```python
from build123d import *

# Parameters (mm, degrees)
BOSS_EXTRUDE1_DEPTH = 10
SKETCH2_R           = 2.5
CUT_EXTRUDE1_DEPTH  = 10
SKETCH3_R           = 11
CUT_EXTRUDE2_DEPTH  = 10
SKETCH4_R           = 2.5
CUT_EXTRUDE3_DEPTH  = 10


with BuildPart() as part:
    # Sketch1 → Boss-Extrude1 (new body)
    with BuildSketch(Plane(origin=(0, 0, 0), x_dir=(0, 0, -1), z_dir=(1, 0, 0))):
        with BuildLine():
            ThreePointArc((-209.31, 0), (0, -209.31), (209.31, 0))
            Line((209.31, 0), (-209.31, 0))
        make_face()
        with BuildLine():
            Line((-209.31, 0), (209.31, 0))
            ThreePointArc((209.31, 0), (0, 209.31), (-209.31, 0))
        make_face()
        with BuildLine():
            Line((-209.31, -224.4), (209.31, -224.4))
            Line((209.31, -224.4), (209.31, 0))
            ThreePointArc((209.31, 0), (0, -209.31), (-209.31, 0))
            Line((-209.31, 0), (-209.31, -224.4))
        make_face()
    extrude(amount=BOSS_EXTRUDE1_DEPTH)

    # Sketch2 → Cut-Extrude1 (cut)
    with BuildSketch(Plane(origin=(10, 0, 0), x_dir=(0, 0, -1), z_dir=(1, 0, 0))):
        with Locations((129.534891246, 129.534891246)):
            Circle(SKETCH2_R)
        with Locations((92.609775132, 92.609775132)):
            Circle(SKETCH2_R)
        with Locations((92.609775132, -92.609775132)):
            Circle(SKETCH2_R)
        with Locations((129.534891246, -129.534891246)):
            Circle(SKETCH2_R)
        with Locations((-92.609775132, -92.609775132)):
            Circle(SKETCH2_R)
        with Locations((-129.534891246, -129.534891246)):
            Circle(SKETCH2_R)
        with Locations((-92.609775132, 92.609775132)):
            Circle(SKETCH2_R)
        with Locations((-129.534891246, 129.534891246)):
            Circle(SKETCH2_R)
    extrude(amount=-CUT_EXTRUDE1_DEPTH, mode=Mode.SUBTRACT)

    # Sketch3 → Cut-Extrude2 (cut)
    with BuildSketch(Plane(origin=(10, 0, 0), x_dir=(0, 0, -1), z_dir=(1, 0, 0))):
        Circle(SKETCH3_R)
    extrude(amount=-CUT_EXTRUDE2_DEPTH, mode=Mode.SUBTRACT)

    # Sketch4 → Cut-Extrude3 (cut)
    with BuildSketch(Plane(origin=(10, 0, 0), x_dir=(0, 0, -1), z_dir=(1, 0, 0))):
        with Locations((-151.806215462, 102.53511129)):
            Circle(SKETCH4_R)
        with Locations(Location((-102.53511129, 151.806215462, 0), (0, 0, 180))):
            Circle(SKETCH4_R)
        with Locations((102.53511129, 151.806215462)):
            Circle(SKETCH4_R)
        with Locations(Location((151.806215462, 102.53511129, 0), (0, 0, 180))):
            Circle(SKETCH4_R)
        with Locations((151.806215462, -102.53511129)):
            Circle(SKETCH4_R)
        with Locations(Location((102.53511129, -151.806215462, 0), (0, 0, 180))):
            Circle(SKETCH4_R)
        with Locations((-102.53511129, -151.806215462)):
            Circle(SKETCH4_R)
        with Locations(Location((-151.806215462, -102.53511129, 0), (0, 0, 180))):
            Circle(SKETCH4_R)
    extrude(amount=-CUT_EXTRUDE3_DEPTH, mode=Mode.SUBTRACT)


solid = part.part
```
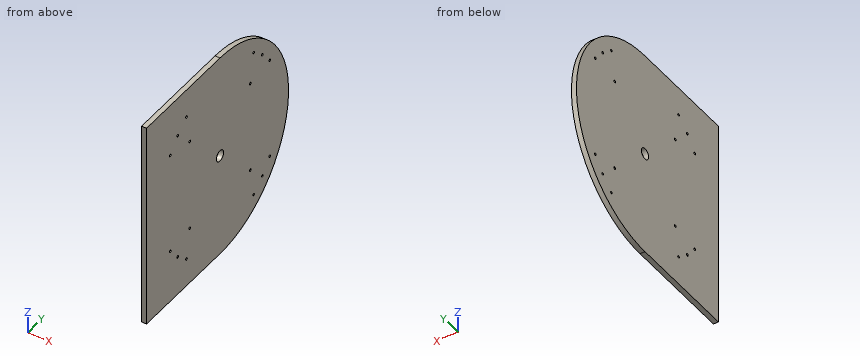
Geometry check sheet. Reference: the model listing, model coordinates, mm. Give positions to 0.01 mm unless a question says otherwise; leave off trailing zeros. Write each loop counter-clockwise with the first axis right and the second up, starting at its lowest first coordinate (ties: lowest second). Pieces come first, ordered by that corner, then holes. Notation, with made-up numbers: (30.5, 54.25) - (88.5, 54.25) arc R20 ccw to (88.5, 89.25) - close; hole circle Ø1 at (46, 59.25). An arc over 180 degrees is marked (long way). Use a Markdown table: item, result.
Q1. Section check A-A, the plane z = 0. Enter the section's corners in (x, y).
Computed:
| item | result |
|---|---|
| outline | (0, -224.4) - (10, -224.4) - (10, -11) - (0, -11) - close; (0, 11) - (10, 11) - (10, 209.31) - (0, 209.31) - close |
Q2. Go/stop test with flat-tipped pins: P1, Ø8, axis at y = -151.81, z = 102.54, coming from the -X side; P2, Ø1, axis at x = 8, y = 94.5, coming from the -Z side; P3, Ø2, axis at x = 1.5, y = 82, coming from the +Z side; P4, Ø5, axis at x = 4, y = 101, coming from the -Z side. Record where each tip stops, or that it passes through.
Computed:
| item | result |
|---|---|
| P1 | stops at x = 0 |
| P2 | stops at z = -187.02 |
| P3 | stops at z = 193 |
| P4 | stops at z = -184.68 |
Q3. Thickness scan on L1, parallel to Y at x = 8.25, z = 128; L2, parallel to Z at x = 8.25, y = -94.5; L3, parallel to Z at x = 8.5, y = 9. Record the ranges inside material, lowest first. Write a range as [from, to].
Computed:
| item | result |
|---|---|
| L1 | y = [-224.4, -131.51], [-127.56, 127.56], [131.51, 165.61] |
| L2 | z = [-209.31, -94.25], [-90.97, 90.97], [94.25, 209.31] |
| L3 | z = [-209.12, -6.32], [6.32, 209.12] |
Q4. Section check B-B, the plane x = 8.5. Give the number of separate pieces and of enclosed holes in the cut face, then the cut area to 3 significant figures.
Computed:
| item | result |
|---|---|
| separate pieces | 1 |
| enclosed holes | 17 |
| area | 162,000 mm² |
Q5. Section check C-C, the plane y = 117.5. Enter the section's corners in (x, z), then the cut area to 3 significant figures.
Computed:
| item | result |
|---|---|
| outline | (0, -173.22) - (10, -173.22) - (10, 173.22) - (0, 173.22) - close |
| area | 3,460 mm² |
